from build123d import *

# Parameters (mm, degrees)
SKETCH1_R           = 2.032
SKETCH1_RX          = 2.032
SKETCH1_RY          = 2.031999502
BOSS_EXTRUDE1_DEPTH = 3.175
FILLET1_R           = 4.7625


with BuildPart() as part:
    # Sketch1 → Boss-Extrude1 (new body)
    with BuildSketch(Plane.XY):
        Polygon((-40.530490432, 38.563534157), (17.380628715, 52.371523419), (26.574151776, 13.813613269), (66.017725223, 13.813613269), (66.017725223, -16.462333503), (-27.410443695, -16.462333503), align=None)
        with Locations((-36.609618565, 36.052645813)):
            Circle(SKETCH1_R, mode=Mode.SUBTRACT)
        with Locations((-30.41013892, 37.427037361)):
            Circle(SKETCH1_R, mode=Mode.SUBTRACT)
        with Locations((-32.967480962, 19.624024753)):
            Circle(SKETCH1_R, mode=Mode.SUBTRACT)
        with Locations((52.87506012, -6.929134334)):
            Circle(SKETCH1_R, mode=Mode.SUBTRACT)
        with Locations((-13.545923607, -6.929134334)):
            Circle(SKETCH1_R, mode=Mode.SUBTRACT)
        with Locations(Location((52.883061118, 5.135865666), (0, 0, 90))):
            Ellipse(SKETCH1_RX, SKETCH1_RY, mode=Mode.SUBTRACT)
        with Locations(Location((-13.537922609, 5.135865666), (0, 0, 90))):
            Ellipse(SKETCH1_RX, SKETCH1_RY, mode=Mode.SUBTRACT)
        with BuildLine():
            ThreePointArc((9.01240199, 27.419307073), (9.31297022, 28.997375114), (8.37364252, 30.300564844))
            ThreePointArc((8.37364252, 30.300564844), (5.345303247, 28.117764523), (9.01240199, 27.419307073))
        make_face(mode=Mode.SUBTRACT)
        with BuildLine():
            ThreePointArc((5.370264386, 43.847928133), (5.670832616, 45.425996173), (4.731504917, 46.729185904))
            ThreePointArc((4.731504917, 46.729185904), (1.703165643, 44.546385582), (5.370264386, 43.847928133))
        make_face(mode=Mode.SUBTRACT)
        with BuildLine():
            ThreePointArc((-3.556986303, 41.868804303), (-0.528647029, 44.051604625), (-4.195745772, 44.750062074))
            ThreePointArc((-4.195745772, 44.750062074), (-4.496314002, 43.171994034), (-3.556986303, 41.868804303))
        make_face(mode=Mode.SUBTRACT)
        with BuildLine():
            ThreePointArc((0.085151301, 25.440183244), (3.113490574, 27.622983565), (-0.553608169, 28.321441014))
            ThreePointArc((-0.553608169, 28.321441014), (-0.854176399, 26.743372974), (0.085151301, 25.440183244))
        make_face(mode=Mode.SUBTRACT)
        with BuildLine():
            ThreePointArc((-25.08473606, 19.860153557), (-24.78416783, 21.438221597), (-25.723495529, 22.741411327))
            ThreePointArc((-25.723495529, 22.741411327), (-28.751834803, 20.558611006), (-25.08473606, 19.860153557))
        make_face(mode=Mode.SUBTRACT)
    extrude(amount=BOSS_EXTRUDE1_DEPTH)

    # Fillet1
    fillet1_edges = [part.edges().sort_by_distance(p)[0] for p in [
        (-40.530490432, 38.563534157, 1.5875),
        (17.380628715, 52.371523419, 1.5875),
        (26.574151776, 13.813613269, 1.5875),
        (66.017725223, 13.813613269, 1.5875),
        (66.017725223, -16.462333503, 1.5875),
        (-27.410443695, -16.462333503, 1.5875),
    ]]
    fillet(fillet1_edges, radius=FILLET1_R)


solid = part.part
Geometry check sheet. Reference: the model listing, model coordinates, mm. A direction names the side the tool comes from. Round coordinates to 2 decimals unless told otherwise and drop trailing zeros. Loops run counter-clockwise (first coordinate to the right, second up) from the corner with the lowest first, then second, coordinate; pieces in that order, holes last. Notation, with made-up numbers: (-2, 43) -> (16, 43) arc R25 cw to (16, 81) -> close; hole circle Ø3 at (-12, 38). An arc over 180 degrees is marked (long way). Answer as a JSON object with one key per item and string values. Group by question number.
Item 1: Cross-section at A-A, the plane z = 1.5. Count the separate pieces of the cut face and the enclosed holes in it, plus the area to 3 significant figures.
Item 2: Release check for a two-part mould opening along X. For faces 1 (the face through (27.348, 14.866, 1.61)), 2 (the face through (-11.915, 45.386, 1.565)), 3 (the face through (-28.472, 38.037, 1.565)) record: pulls with the +X half, pulls with the -X half, needs draft (parallel to the pull), parting line crosses it, or undercut.
Item 3: Depth check by flat-ended pin: pin 1 Ø5.5 at (x, y) = (-36.61, 36.05) entering from -Z. Enter the tip coordinate at first touch or a pass-through.
Item 4: Set-up check for faces 4 (the face through (50.845, -6.84, 1.565)), 5 (the face through (46, 13.814, 2)): record each of +Z, -Z, +X, -X, +Y, -Y from which the full face is reachable in a straight line by a thin tool's end or side.
Item 5: Thickness scan on line 1 along Y through (x, z) = (-14, 0.3); line 2 along X through (y, z) = (20.5, 1.85); line 3 along Y through (x, z) = (61.5, 0.3). Record the ranges inside material, lowest first.
Item 6: Cross-section at B-B, the plane x = 57. Record the cut outline in (y, z) (3 decimals), plus the area to 3 significant figures.
Determined:
{
 "1": {"separate pieces": "1", "enclosed holes": "12", "area": "4,700 mm²"},
 "2": {"face 1": "pulls with the +X half", "face 2": "pulls with the -X half", "face 3": "undercut"},
 "3": {"pin 1": "stops at z = 0"},
 "4": {"face 4": "+Z, -Z", "face 5": "+Z, -Z, +X, +Y"},
 "5": {"line 1": "y = -16.46 to -8.91, -4.95 to 3.16, 7.11 to 44.89", "line 2": "x = -36.22 to -34.8, -31.13 to -28.74, -24.8 to 24.98", "line 3": "y = -16.46 to 13.81"},
 "6": {"outline": "(-16.462, 0) -> (13.814, 0) -> (13.814, 3.175) -> (-16.462, 3.175) -> close", "area": "96.1 mm²"}
}
